```python
from build123d import *

# Parameters (mm, degrees)
SKETCH1_W               = 69
SKETCH1_H               = 32
BOSS_EXTRUDE1_DEPTH     = 2
SKETCH2_W               = 69
SKETCH2_H               = 32
SKETCH2_W_2             = 63
SKETCH2_H_2             = 26
BOSS_EXTRUDE2_DEPTH     = 6
SKETCH3_R               = 2.5
SKETCH3_R_2             = 1.5
BOSS_EXTRUDE3_DEPTH     = 2
CUT_EXTRUDE1_DEPTH      = 39.5
CUT_EXTRUDE1_DEPTH_BACK = 39.5
SKETCH4_R               = 1.5
SKETCH4_W               = 10.4
SKETCH4_H               = 8


with BuildPart() as part:
    # Sketch1 → Boss-Extrude1 (new body)
    with BuildSketch(Plane.XY):
        Rectangle(SKETCH1_W, SKETCH1_H)
    extrude(amount=BOSS_EXTRUDE1_DEPTH)

    # Sketch2 → Boss-Extrude2 (add)
    with BuildSketch(Plane.XY.offset(2)):
        Rectangle(SKETCH2_W, SKETCH2_H)
        Rectangle(SKETCH2_W_2, SKETCH2_H_2, mode=Mode.SUBTRACT)
    extrude(amount=BOSS_EXTRUDE2_DEPTH)

    # Sketch3 → Boss-Extrude3 (add)
    # profile 1 of 6: a face of its own
    with BuildSketch(Plane.XY.offset(2)):
        with Locations((-28, 9.5)):
            Circle(SKETCH3_R)
        with Locations((-28, 9.5)):
            Circle(SKETCH3_R_2, mode=Mode.SUBTRACT)
    # profile 2 of 6: a face of its own
    with BuildSketch(Plane.XY.offset(2)):
        with Locations((-28, -9.5)):
            Circle(SKETCH3_R)
        with Locations((-28, -9.5)):
            Circle(SKETCH3_R_2, mode=Mode.SUBTRACT)
    # profile 3 of 6: a face of its own
    with BuildSketch(Plane.XY.offset(2)):
        with Locations((28, -9.5)):
            Circle(SKETCH3_R)
        with Locations((28, -9.5)):
            Circle(SKETCH3_R_2, mode=Mode.SUBTRACT)
    # profile 4 of 6: a face of its own
    with BuildSketch(Plane.XY.offset(2)):
        with Locations((28, 9.5)):
            Circle(SKETCH3_R)
        with Locations((28, 9.5)):
            Circle(SKETCH3_R_2, mode=Mode.SUBTRACT)
    # profile 5 of 6: a face of its own
    with BuildSketch(Plane.XY.offset(2)):
        with Locations((-7, 0)):
            Circle(SKETCH3_R)
    # profile 6 of 6: a face of its own
    with BuildSketch(Plane.XY.offset(2)):
        with Locations((7, 0)):
            Circle(SKETCH3_R)
    extrude(amount=BOSS_EXTRUDE3_DEPTH)

    # Sketch4 → Cut-Extrude1 (cut, two sides: drawn at the far end of the back side and taken through both)
    with BuildSketch(Plane.XY.offset(2).offset(-CUT_EXTRUDE1_DEPTH_BACK)):
        with Locations((28, 9.5)):
            Circle(SKETCH4_R)
        with Locations((28, -9.5)):
            Circle(SKETCH4_R)
        with Locations((-28, -9.5)):
            Circle(SKETCH4_R)
        with Locations((-28, 9.5)):
            Circle(SKETCH4_R)
        with Locations((-20.6, -9)):
            Rectangle(SKETCH4_W, SKETCH4_H)
        with Locations((-7.6, -9)):
            Rectangle(SKETCH4_W, SKETCH4_H)
        with Locations((7.6, -9)):
            Rectangle(SKETCH4_W, SKETCH4_H)
        with Locations((20.6, -9)):
            Rectangle(SKETCH4_W, SKETCH4_H)
    extrude(amount=CUT_EXTRUDE1_DEPTH + CUT_EXTRUDE1_DEPTH_BACK, mode=Mode.SUBTRACT)


solid = part.part
```
Verification items for the finished model (mm, model axes). A direction names the side the tool comes from. Give positions to 0.01 mm unless a question says otherwise; leave off trailing zeros. Loops run counter-clockwise (first coordinate to the right, second up) from the corner with the lowest first, then second, coordinate; pieces in that order, holes last.
1. Section check B-B, the plane y = 9.5. Enter the section's corners in (x, z), then the cut area to 3 significant figures.
2. Section check D-D, the plane y = -6. Enter the section's corners in (x, z).
3. Mould release check, pull along X, two halves, no side actions. Record for faces 1 (the flat face through (21, -5, 1)), 2 (the flat face through (0, -16, 4)), 3 (the flat face through (-12.8, -9, 1)), 4 (the flat face through (-34.5, 0, 4)): released by +X, released by -X, zero draft, split by the parting line, or undercut.
4. Section check A-A, the plane x = 28. Enter the section's corners in (y, z), then the cut area to 3 significant figures.
5. Set-up check for faces 5 (the flat face through (25.8, -9, 2)), 6 (the flat face through (34.5, 0, 4)), 7 (the cylindrical face through (27.46, 7.06, 2.99)): record each of +Z, -Z, +X, -X, +Y, -Y from which the full face is reachable in a straight line by a thin tool's end or side.
6. Section check C-C, the plane x = -19.5. Enter the section's corners in (y, z), then the cut area to 3 significant figures.
7. Go/stop test with flat-tipped pins: pin 1 Ø2 at (x, y) = (2.5, -8) entering from +Z; pin 2 Ø2.5 at (x, y) = (-8, 0.5) entering from +Z; pin 3 Ø4 at (x, y) = (-28, -9.5) entering from -Z. Record where each tip stops, or that it passes through.
8. Thickness scan on line 1 (Y direction, x = -28, z = 1.4); line 2 (Y direction, x = 28, z = 2.75); line 3 (Y direction, x = -28, z = 5.5). Record the ranges inside material, lowest first.
Geometry says:
1. outline: (-34.5, 0) - (-29.5, 0) - (-29.5, 4) - (-30.5, 4) - (-30.5, 2) - (-31.5, 2) - (-31.5, 8) - (-34.5, 8) - close; (-26.5, 0) - (26.5, 0) - (26.5, 4) - (25.5, 4) - (25.5, 2) - (-25.5, 2) - (-25.5, 4) - (-26.5, 4) - close; (29.5, 0) - (34.5, 0) - (34.5, 8) - (31.5, 8) - (31.5, 2) - (30.5, 2) - (30.5, 4) - (29.5, 4) - close
1. area: 170 mm2
2. outline: (-34.5, 0) - (-25.8, 0) - (-25.8, 2) - (-31.5, 2) - (-31.5, 8) - (-34.5, 8) - close; (-15.4, 0) - (-12.8, 0) - (-12.8, 2) - (-15.4, 2) - close; (-2.4, 0) - (2.4, 0) - (2.4, 2) - (-2.4, 2) - close; (12.8, 0) - (15.4, 0) - (15.4, 2) - (12.8, 2) - close; (25.8, 0) - (34.5, 0) - (34.5, 8) - (31.5, 8) - (31.5, 2) - (25.8, 2) - close
3. face 1: undercut
3. face 2: zero draft
3. face 3: undercut
3. face 4: released by -X
4. outline: (-16, 0) - (-11, 0) - (-11, 4) - (-12, 4) - (-12, 2) - (-13, 2) - (-13, 8) - (-16, 8) - close; (-8, 0) - (8, 0) - (8, 4) - (7, 4) - (7, 2) - (-7, 2) - (-7, 4) - (-8, 4) - close; (11, 0) - (16, 0) - (16, 8) - (13, 8) - (13, 2) - (12, 2) - (12, 4) - (11, 4) - close
4. area: 96.0 mm2
5. face 5: +Z, -Z
5. face 6: +Z, -Z, +X, +Y, -Y
5. face 7: +Z
6. outline: (-16, 0) - (-13, 0) - (-13, 8) - (-16, 8) - close; (-5, 0) - (16, 0) - (16, 8) - (13, 8) - (13, 2) - (-5, 2) - close
6. area: 84.0 mm2
7. pin 1: stops at z = 2
7. pin 2: stops at z = 4
7. pin 3: stops at z = 0
8. line 1: y = -16 to -11, -8 to 8, 11 to 16
8. line 2: y = -16 to -13, -12 to -11, -8 to -7, 7 to 8, 11 to 12, 13 to 16
8. line 3: y = -16 to -13, 13 to 16
